Autodesk Inventor part; units mm, degrees
ref_plane "YZ Plane" through (0, 0, 0) normal (1, 0, 0) x (0, 1, 0)
ref_plane "XZ Plane" through (0, 0, 0) normal (0, 1, 0) x (-1, 0, 0)
ref_plane "XY Plane" through (0, 0, 0) normal (0, 0, 1) x (1, 0, 0)
sketch "Schizzo1" plane through (0, 0, 0) normal (1, 0, 0) x (0, 1, 0)
  line L0 (0, 0) -> (25, 0)
  line L1 (25, 0) -> (0, -16)
  line L2 (0, -16) -> (0, 0)
  dimension "d0" = 16
  dimension "d1" = 25
extrude "Estrusione1" add sketch "Schizzo1" along normal blind 4
sketch "Schizzo2" plane through (4, 0, 0) normal (1, 0, 0) x (0, 0, -1)
  line L0 (0, 0) -> (16, 0)
  line L1 (16, 0) -> (11, 0)
  line L2 (11, 0) -> (11, -4)
  line L3 (11, -4) -> (16, -4)
  line L4 (16, -4) -> (16, 0)
  line L5 (11, 0) -> (6, 0)
  line L6 (6, 0) -> (1, 0)
  line L7 (1, 0) -> (1, -4)
  line L8 (1, -4) -> (6, -4)
  line L9 (6, -4) -> (6, 0)
  line L10 (0, 25) -> (0, 0)
  line L11 (0, 0) -> (0, 5)
  line L12 (0, 5) -> (-4, 5)
  line L13 (-4, 5) -> (-4, 0)
  line L14 (-4, 0) -> (0, 0)
  line L15 (0, 15) -> (-4, 15)
  line L16 (-4, 15) -> (-4, 10)
  line L17 (-4, 10) -> (0, 10)
  line L18 (0, 10) -> (0, 15)
  line L19 (0, 25) -> (-4, 25)
  line L20 (-4, 25) -> (-4, 20)
  line L21 (-4, 20) -> (0, 20)
  line L22 (0, 20) -> (0, 25)
  dimension "d4" = 5
  dimension "d5" = 4
  dimension "d6" = 5
  dimension "d7" = 5
  dimension "d8" = 4
  dimension "d9" = 5
  dimension "d10" = 4
  dimension "d13" = 10
extrude "Estrusione2" add sketch "Schizzo2" against normal blind 4
properties part number "laterali"
The model under review builds one solid part; all positions refer to its coordinate system, in mm. A direction names the side the tool comes from. Coordinates: 2 decimals unless noted, no trailing zeros. Order: outer loops, then holes, each group sorted by start corner. A loop starts at its lowest first (then second) coordinate and runs counter-clockwise, first axis right, second up. Notation, with made-up numbers: (4, -22) -> (48, -22) arc R11 cw to (48, -16) -> close; hole circle Ø9 at (-28, 11.25). An arc over 180 degrees is marked (long way). Answer in a Markdown table with one row per item. Add a question column.
Item 1: We need section A-A on y = -0.75. Write out the cut boundary in (x, z).
Item 2: We need section B-B on x = 1.65. Write out the cut boundary in (y, z), plus the area to 3 significant figures.
Item 3: We need section D-D on y = 16. Write out the cut boundary in (x, z).
Item 4: Machinability: for faces 1 (the flat face through (2, 0, -9)), 2 (the flat face through (2, -2, -1)), 3 (the flat face through (2, 7, 0)), which of the approach directions +Z, -Z, +X, -X, +Y, -Y give a long, thin tool a straight path to every point of the face, cutting with its end or side? Answer none if there is none.
Item 5: To check wall thickness, follow probe 1 along Y at (x, z) = (3.6, 1); probe 2 along Z at (x, y) = (3, -0.5); probe 3 along Y at (x, z) = (1.7, -5.5). State the ranges of each line that lie inside material, in increasing order.
Item 6: We need section C-C on z = 1. Write out the cut boundary in (x, y).
Item 7: Clearance check with flat-ended pins moving along their axes: pin 1 (6 mm diameter, centred on y = 7.5, z = -4.5, fed in from -X); pin 2 (1 mm diameter, centred on x = 0.5, z = -3, fed in from +Y); pin 3 (1.2 mm diameter, centred on x = 2.5, z = 1.5, fed in from -Y); pin 4 (2 mm diameter, centred on x = 0.5, z = -14, fed in from +Y). State where each tip first meets the part, or that it passes through.
Item 8: Mouldability with a two-part tool opening along Z and no side actions: class faces 4 (the flat face through (2, -2, -6)), 5 (the flat face through (1.97, 12.67, -7.89)), 6 (the flat face through (2, 25, 2)) as +Z half, -Z half, draft (parallel to the pull), parting line (faces both ways), or undercut.
Final values:
| question | item | result |
|---|---|---|
| 1 | outline | (0, -16) -> (4, -16) -> (4, -11) -> (0, -11) -> close; (0, -6) -> (4, -6) -> (4, -1) -> (0, -1) -> close |
| 2 | outline | (-4, -16) -> (0, -16) -> (25, 0) -> (25, 4) -> (20, 4) -> (20, 0) -> (15, 0) -> (15, 4) -> (10, 4) -> (10, 0) -> (5, 0) -> (5, 4) -> (0, 4) -> (0, -1) -> (-4, -1) -> (-4, -6) -> (0, -6) -> (0, -11) -> (-4, -11) -> close |
| 2 | area | 300 mm2 |
| 3 | outline | (0, -5.76) -> (4, -5.76) -> (4, 0) -> (0, 0) -> close |
| 4 | face 1 | +X, -X, -Y |
| 4 | face 2 | +Z, +X, -X, -Y |
| 4 | face 3 | +Z, +X, -X |
| 5 | probe 1 | y = 0 to 5, 10 to 15, 20 to 25 |
| 5 | probe 2 | z = -16 to -11, -6 to -1 |
| 5 | probe 3 | y = -4 to 16.41 |
| 6 | outline | (0, 0) -> (4, 0) -> (4, 5) -> (0, 5) -> close; (0, 10) -> (4, 10) -> (4, 15) -> (0, 15) -> close; (0, 20) -> (4, 20) -> (4, 25) -> (0, 25) -> close |
| 7 | pin 1 | stops at x = 0 |
| 7 | pin 2 | stops at y = 21.09 |
| 7 | pin 3 | stops at y = 0 |
| 7 | pin 4 | stops at y = 4.69 |
| 8 | face 4 | undercut |
| 8 | face 5 | -Z half |
| 8 | face 6 | draft |
